Can you work these out from the model? Positions are in its coordinate system, mm. A direction names the side the tool comes from. Coordinates: 2 decimals unless noted, no trailing zeros. Order: outer loops, then holes, each group sorted by start corner. A loop starts at its lowest first (then second) coordinate and runs counter-clockwise, first axis right, second up. Notation, with made-up numbers: M -28,33.25 L -23,33.25 A21 ccw -23,43.25 Z; hole C 30.5,41.5 d5. An arc over 180 degrees is marked long. Answer as a JSON object with one key per item and string values.
from build123d import *

# Parameters (mm, degrees)
SKETCH1_R           = 6.55
BOSS_EXTRUDE1_DEPTH = 1.35
SKETCH2_W           = 0.7
SKETCH2_H           = 3.730882663
SKETCH2_W_2         = 1.5
SKETCH2_H_2         = 13.460629035
BOSS_EXTRUDE2_DEPTH = 9.2
SKETCH3_W           = 1.5
SKETCH3_H           = 13.1
SKETCH3_W_2         = 0.65
SKETCH3_H_2         = 5
BOSS_EXTRUDE3_DEPTH = 1
CUT_EXTRUDE1_DEPTH  = 29.3
CUT_EXTRUDE2_DEPTH  = 45.6
SKETCH7_W           = 41.6
SKETCH7_H           = 7
BOSS_EXTRUDE4_DEPTH = 0.5
SKETCH8_R           = 0.4
PINS_DEPTH          = 11
PINS_2_DEPTH        = 11
PINS_3_DEPTH        = 11
PINS_4_DEPTH        = 11
PINS_5_DEPTH        = 11
PINS_6_DEPTH        = 11
PINS_7_DEPTH        = 11
PINS_8_DEPTH        = 11
SKETCH9_W           = 2.08
SKETCH9_H           = 2.08
BOSS_EXTRUDE6_DEPTH = 11


with BuildPart() as part:
    # Sketch1 → Boss-Extrude1 (new body)
    with BuildSketch(Plane.XY):
        with BuildLine():
            Line((0, 8), (-4, 8))
            Line((-4, 8), (-4, 13.989370965))
            ThreePointArc((-4, 13.989370965), (-8.760779075, -11.616851983), (14.55, 0))
            ThreePointArc((14.55, 0), (11.616851983, 8.760779075), (4, 13.989370965))
            Line((4, 13.989370965), (4, 8))
            Line((4, 8), (0, 8))
        make_face()
        Circle(SKETCH1_R, mode=Mode.SUBTRACT)
    extrude(amount=BOSS_EXTRUDE1_DEPTH)

    # Sketch2 → Boss-Extrude2 (add)
    with BuildSketch(Plane.XY.offset(1.35)):
        with BuildLine():
            ThreePointArc((12.120231021, 8.05), (12.578647446, 7.313010901), (12.992305415, 6.55))
            Line((12.992305415, 6.55), (22.3, 6.55))
            Line((22.3, 6.55), (22.3, 8.05))
            Line((22.3, 8.05), (12.120231021, 8.05))
        make_face()
        with Locations((5.65, 9.915441332)):
            Rectangle(SKETCH2_W, SKETCH2_H)
        with BuildLine():
            Line((-5.3, 8.05), (-6, 8.05))
            Line((-6, 8.05), (-12.120231021, 8.05))
            ThreePointArc((-12.120231021, 8.05), (-12.578647446, 7.313010901), (-12.992305415, 6.55))
            Line((-12.992305415, 6.55), (12.992305415, 6.55))
            ThreePointArc((12.992305415, 6.55), (12.578647446, 7.313010901), (12.120231021, 8.05))
            Line((12.120231021, 8.05), (6, 8.05))
            Line((6, 8.05), (5.3, 8.05))
            Line((5.3, 8.05), (4, 8.05))
            Line((4, 8.05), (4, 8))
            Line((4, 8), (-4, 8))
            Line((-4, 8), (-4, 8.05))
            Line((-4, 8.05), (-5.3, 8.05))
        make_face()
        with BuildLine():
            ThreePointArc((-12.992305415, 6.55), (-12.578647446, 7.313010901), (-12.120231021, 8.05))
            Line((-12.120231021, 8.05), (-22.3, 8.05))
            Line((-22.3, 8.05), (-22.3, 6.55))
            Line((-22.3, 6.55), (-12.992305415, 6.55))
        make_face()
        with Locations((-21.55, -14.780314518)):
            Rectangle(SKETCH2_W_2, SKETCH2_H_2)
        with BuildLine():
            ThreePointArc((-12.120231021, -8.05), (-12.578647446, -7.313010901), (-12.992305415, -6.55))
            Line((-12.992305415, -6.55), (-22.3, -6.55))
            Line((-22.3, -6.55), (-22.3, -8.05))
            Line((-22.3, -8.05), (-20.8, -8.05))
            Line((-20.8, -8.05), (-12.120231021, -8.05))
        make_face()
        with BuildLine():
            Line((12.992305415, -6.55), (-12.992305415, -6.55))
            ThreePointArc((-12.992305415, -6.55), (-12.578647446, -7.313010901), (-12.120231021, -8.05))
            Line((-12.120231021, -8.05), (12.120231021, -8.05))
            ThreePointArc((12.120231021, -8.05), (12.578647446, -7.313010901), (12.992305415, -6.55))
        make_face()
        with BuildLine():
            Line((22.3, -6.55), (12.992305415, -6.55))
            ThreePointArc((12.992305415, -6.55), (12.578647446, -7.313010901), (12.120231021, -8.05))
            Line((12.120231021, -8.05), (20.8, -8.05))
            Line((20.8, -8.05), (22.3, -8.05))
            Line((22.3, -8.05), (22.3, -6.55))
        make_face()
        with Locations((21.55, -14.780314518)):
            Rectangle(SKETCH2_W_2, SKETCH2_H_2)
        with Locations((-5.65, 9.915441332)):
            Rectangle(SKETCH2_W, SKETCH2_H)
    extrude(amount=BOSS_EXTRUDE2_DEPTH)

    # Sketch3 → Boss-Extrude3 (add)
    with BuildSketch(Plane.XY.offset(1.35)):
        with Locations((-20.9, 0)):
            Rectangle(SKETCH3_W, SKETCH3_H)
        with Locations((-21.975, 0)):
            Rectangle(SKETCH3_W_2, SKETCH3_H_2)
        with Locations((21.975, 0)):
            Rectangle(SKETCH3_W_2, SKETCH3_H_2)
        with Locations((20.9, 0)):
            Rectangle(SKETCH3_W, SKETCH3_H)
    extrude(amount=BOSS_EXTRUDE3_DEPTH)

    # Sketch5 → Cut-Extrude1 (cut, through all)
    with BuildSketch(Plane(origin=(6, 0, 0), x_dir=(0, 0, -1), z_dir=(1, 0, 0))):
        Polygon((-10.55, 8.05), (-5.080882663, 8.05), (-1.35, 11.780882663), (-10.55, 11.780882663), align=None)
    extrude(amount=-CUT_EXTRUDE1_DEPTH, mode=Mode.SUBTRACT)

    # Sketch6 → Cut-Extrude2 (cut, through all)
    with BuildSketch(Plane(origin=(22.3, 0, 0), x_dir=(0, 0, -1), z_dir=(1, 0, 0))):
        Polygon((-7.55, -21.510629035), (-7.55, -17.317508604), (-4.282491396, -14.05), (-1.35, -14.05), (-1.35, -21.510629035), align=None)
    extrude(amount=-CUT_EXTRUDE2_DEPTH, mode=Mode.SUBTRACT)

    # Sketch7 → Boss-Extrude4 (add)
    with BuildSketch(Plane.XY.offset(1.35)):
        with Locations((0, -11.55)):
            Rectangle(SKETCH7_W, SKETCH7_H)
    extrude(amount=BOSS_EXTRUDE4_DEPTH)



with BuildPart() as body_2:
    # Sketch8 → Pins (new body)
    with BuildSketch(Plane.XZ.offset(15.05)):
        with Locations((-17.78, 2.39)):
            Circle(SKETCH8_R)
    extrude(amount=PINS_DEPTH)


with BuildPart() as body_3:
    # Sketch8 → Pins 2 (new body)
    with BuildSketch(Plane.XZ.offset(15.05)):
        with Locations((-12.7, 2.39)):
            Circle(SKETCH8_R)
    extrude(amount=PINS_2_DEPTH)


with BuildPart() as body_4:
    # Sketch8 → Pins 3 (new body)
    with BuildSketch(Plane.XZ.offset(15.05)):
        with Locations((-7.62, 2.39)):
            Circle(SKETCH8_R)
    extrude(amount=PINS_3_DEPTH)


with BuildPart() as body_5:
    # Sketch8 → Pins 4 (new body)
    with BuildSketch(Plane.XZ.offset(15.05)):
        with Locations((-2.54, 2.39)):
            Circle(SKETCH8_R)
    extrude(amount=PINS_4_DEPTH)


with BuildPart() as body_6:
    # Sketch8 → Pins 5 (new body)
    with BuildSketch(Plane.XZ.offset(15.05)):
        with Locations((2.54, 2.39)):
            Circle(SKETCH8_R)
    extrude(amount=PINS_5_DEPTH)


with BuildPart() as body_7:
    # Sketch8 → Pins 6 (new body)
    with BuildSketch(Plane.XZ.offset(15.05)):
        with Locations((7.62, 2.39)):
            Circle(SKETCH8_R)
    extrude(amount=PINS_6_DEPTH)


with BuildPart() as body_8:
    # Sketch8 → Pins 7 (new body)
    with BuildSketch(Plane.XZ.offset(15.05)):
        with Locations((12.7, 2.39)):
            Circle(SKETCH8_R)
    extrude(amount=PINS_7_DEPTH)


with BuildPart() as body_9:
    # Sketch8 → Pins 8 (new body)
    with BuildSketch(Plane.XZ.offset(15.05)):
        with Locations((17.78, 2.39)):
            Circle(SKETCH8_R)
    extrude(amount=PINS_8_DEPTH)


with BuildPart() as part_1:
    add(part.part)

    add(body_2.part)  # Boss-Extrude6 merges body 2

    add(body_3.part)  # Boss-Extrude6 merges body 3

    add(body_4.part)  # Boss-Extrude6 merges body 4

    add(body_5.part)  # Boss-Extrude6 merges body 5

    add(body_6.part)  # Boss-Extrude6 merges body 6

    add(body_7.part)  # Boss-Extrude6 merges body 7

    add(body_8.part)  # Boss-Extrude6 merges body 8

    add(body_9.part)  # Boss-Extrude6 merges body 9
    # Sketch9 → Boss-Extrude6 (add)
    with BuildSketch(Plane.XZ.offset(8.05)):
        with Locations((-12.7, 2.39)):
            Rectangle(SKETCH9_W, SKETCH9_H)
        with Locations((-17.78, 2.39)):
            Rectangle(SKETCH9_W, SKETCH9_H)
        with Locations((-7.62, 2.39)):
            Rectangle(SKETCH9_W, SKETCH9_H)
        with Locations((-2.54, 2.39)):
            Rectangle(SKETCH9_W, SKETCH9_H)
        with Locations((2.54, 2.39)):
            Rectangle(SKETCH9_W, SKETCH9_H)
        with Locations((7.62, 2.39)):
            Rectangle(SKETCH9_W, SKETCH9_H)
        with Locations((12.7, 2.39)):
            Rectangle(SKETCH9_W, SKETCH9_H)
        with Locations((17.78, 2.39)):
            Rectangle(SKETCH9_W, SKETCH9_H)
    extrude(amount=BOSS_EXTRUDE6_DEPTH)


solid = part_1.part
Item 1: I'm going to push flat-ended pins straight in: pin 1 (10 mm diameter, centred on x = -8, y = -2, fed in from -Z); pin 2 (1 mm diameter, centred on x = -2, y = -12, fed in from +Z); pin 3 (1.7 mm diameter, centred on y = -15, z = 2, fed in from -X); pin 4 (4 mm diameter, centred on y = -20.5, z = 2.5, fed in from -X). Where does each tip first touch, or does it pass through?
Answers follow:
{"pin 1": "stops at z = 0", "pin 2": "stops at z = 3.43", "pin 3": "stops at x = -20.8", "pin 4": "stops at x = -18.82"}
Item 2: Please list where these lines run through material, in increasing order: line 1 (Y direction, x = -1, z = 5.5); line 2 (Y direction, x = 0, z = 0.95); line 3 (X direction, y = 0, z = 0.7).
Answers follow:
{"line 1": "y = -8.05 to -6.55, 6.55 to 8", "line 2": "y = -14.55 to -6.55, 6.55 to 8", "line 3": "x = -14.55 to -6.55, 6.55 to 14.55"}
Item 3: If we mould it in two halves opening along Y, with no side actions, what happens to faces 1 (the flat face through (20.15, 0, 2)), 2 (the flat face through (13, -19.05, 3)), 3 (the flat face through (-3.4, -14.5, 1.35))? For each: pulls with the +Y half, pulls with the -Y half, needs draft (parallel to the pull), parting line crosses it, or undercut.
Answers follow:
{"face 1": "undercut", "face 2": "pulls with the -Y half", "face 3": "needs draft"}
Item 4: I want a section at D-D, the plane y = 10.5. Write out the boundary of the cut face in (x, z), plus the area to 3 significant figures.
Answers follow:
{"outline": "M -10.07,0 L -4,0 L -4,1.35 L -5.3,1.35 L -5.3,2.63 L -6,2.63 L -6,1.35 L -10.07,1.35 Z; M 4,0 L 10.07,0 L 10.07,1.35 L 6,1.35 L 6,2.63 L 5.3,2.63 L 5.3,1.35 L 4,1.35 Z", "area": "18.2 mm^2"}
Item 5: I want a section at B-B, the plane z = 9. Write out the boundary of the cut face in (x, y).
Answers follow:
{"outline": "M -22.3,-21.51 L -20.8,-21.51 L -20.8,-8.05 L 20.8,-8.05 L 20.8,-21.51 L 22.3,-21.51 L 22.3,-6.55 L -22.3,-6.55 Z; M -22.3,6.55 L 22.3,6.55 L 22.3,8.05 L 4,8.05 L 4,8 L -4,8 L -4,8.05 L -22.3,8.05 Z"}
Item 6: Which directions (+Z, -Z, +X, -X, +Y, -Y) give clear straight access to the entire face, cutting with the end or side of a thin tool? Please do faces 4 (the flat face through (6, 9, 3)), 5 (the flat face through (3.58, -13, 3)), 6 (the flat face through (4, 11, 1)).
Answers follow:
{"face 4": "+Z, +X, +Y", "face 5": "+Z, -Y", "face 6": "+Z, -Z, +Y"}
Item 7: I want a section at C-C, the plane y = 1.5. Write out the boundary of the cut face in (x, z), plus the area to 3 significant figures.
Answers follow:
{"outline": "M -22.3,1.35 L -20.15,1.35 L -20.15,2.35 L -22.3,2.35 Z; M -14.47,0 L -6.38,0 L -6.38,1.35 L -14.47,1.35 Z; M 6.38,0 L 14.47,0 L 14.47,1.35 L 6.38,1.35 Z; M 20.15,1.35 L 22.3,1.35 L 22.3,2.35 L 20.15,2.35 Z", "area": "26.2 mm^2"}
Item 8: I want a section at A-A, the plane y = -22.5. Write out the boundary of the cut face in (x, z).
Answers follow:
{"outline": "C -17.78,2.39 d0.8; C -12.7,2.39 d0.8; C -7.62,2.39 d0.8; C -2.54,2.39 d0.8; C 2.54,2.39 d0.8; C 7.62,2.39 d0.8; C 12.7,2.39 d0.8; C 17.78,2.39 d0.8"}
